from build123d import *

# Parameters (mm, degrees)
SKETCH1_R                = 7.5
BOSS_EXTRUDE1_DEPTH      = 15
BOSS_EXTRUDE2_DEPTH      = 45
BOSS_EXTRUDE3_DEPTH      = 18
BOSS_EXTRUDE3_DEPTH_BACK = 15
CUT_EXTRUDE1_REACH       = 187.068
SKETCH2_R                = 4
CUT_EXTRUDE2_REACH       = 188.456
SKETCH3_R                = 5


with BuildPart() as part:
    # Sketch1 → Boss-Extrude1 (new, symmetric)
    with BuildSketch(Plane.XY):
        with BuildLine():
            Line((145, 15), (80, 15))
            Line((80, 15), (80, 0))
            Line((80, 0), (175, 0))
            Line((175, 0), (175, 31))
            ThreePointArc((175, 31), (160, 46), (145, 31))
            Line((145, 31), (145, 15))
        make_face()
        with Locations((160, 31)):
            Circle(SKETCH1_R, mode=Mode.SUBTRACT)
    extrude(amount=BOSS_EXTRUDE1_DEPTH, both=True)



with BuildPart() as body_2:
    # Sketch1_3 → Boss-Extrude2 (new, symmetric)
    with BuildSketch(Plane.XY):
        Polygon((65, 15), (0, 15), (0, -25), (16, -25), (16, 0), (80, 0), align=None)
    extrude(amount=BOSS_EXTRUDE2_DEPTH, both=True)


with BuildPart() as part_1:
    add(part.part)

    add(body_2.part)  # Boss-Extrude3 merges body 2
    # Sketch1_4 → Boss-Extrude3 (add, two sides: drawn at the far end of the back side and taken through both)
    with BuildSketch(Plane.XY.offset(-BOSS_EXTRUDE3_DEPTH_BACK)):
        Polygon((80, 15), (65, 15), (80, 0), align=None)
    extrude(amount=BOSS_EXTRUDE3_DEPTH + BOSS_EXTRUDE3_DEPTH_BACK)

    # Sketch2 → Cut-Extrude1 (cut, up to next)
    with BuildSketch(Plane(origin=(0, 15, 0), x_dir=(1, 0, 0), z_dir=(0, 1, 0)), mode=Mode.PRIVATE) as cut_extrude1_sk1:
        with Locations(Location((55, 0, 0), (0, 0, 180))):
            Circle(SKETCH2_R)
    cut_extrude1_tool1 = extrude(cut_extrude1_sk1.sketch, amount=-CUT_EXTRUDE1_REACH, mode=Mode.PRIVATE) & part_1.part
    # Sketch2 → Cut-Extrude1 (cut, up to next)
    with BuildSketch(Plane(origin=(0, 15, 0), x_dir=(1, 0, 0), z_dir=(0, 1, 0)), mode=Mode.PRIVATE) as cut_extrude1_sk2:
        with Locations(Location((30, 0, 0), (0, 0, 180))):
            Circle(SKETCH2_R)
    cut_extrude1_tool2 = extrude(cut_extrude1_sk2.sketch, amount=-CUT_EXTRUDE1_REACH, mode=Mode.PRIVATE) & part_1.part
    add(cut_extrude1_tool1.solids().sort_by_distance((55, 15, 0))[0], mode=Mode.SUBTRACT)
    add(cut_extrude1_tool2.solids().sort_by_distance((30, 15, 0))[0], mode=Mode.SUBTRACT)

    # Sketch3 → Cut-Extrude2 (cut, up to next)
    with BuildSketch(Plane.ZY, mode=Mode.PRIVATE) as cut_extrude2_sk1:
        with Locations(Location((35, -15, 0), (0, 0, 270))):
            Circle(SKETCH3_R)
    cut_extrude2_tool1 = extrude(cut_extrude2_sk1.sketch, amount=-CUT_EXTRUDE2_REACH, mode=Mode.PRIVATE) & part_1.part
    # Sketch3 → Cut-Extrude2 (cut, up to next)
    with BuildSketch(Plane.ZY, mode=Mode.PRIVATE) as cut_extrude2_sk2:
        with BuildLine():
            Line((45, -25), (45, -15))
            ThreePointArc((45, -15), (42.071067812, -22.071067812), (35, -25))
            Line((35, -25), (45, -25))
        make_face()
    cut_extrude2_tool2 = extrude(cut_extrude2_sk2.sketch, amount=-CUT_EXTRUDE2_REACH, mode=Mode.PRIVATE) & part_1.part
    # Sketch3 → Cut-Extrude2 (cut, up to next)
    with BuildSketch(Plane.ZY, mode=Mode.PRIVATE) as cut_extrude2_sk3:
        with Locations(Location((-35, -15, 0), (0, 0, 270))):
            Circle(SKETCH3_R)
    cut_extrude2_tool3 = extrude(cut_extrude2_sk3.sketch, amount=-CUT_EXTRUDE2_REACH, mode=Mode.PRIVATE) & part_1.part
    # Sketch3 → Cut-Extrude2 (cut, up to next)
    with BuildSketch(Plane.ZY, mode=Mode.PRIVATE) as cut_extrude2_sk4:
        with BuildLine():
            Line((-45, -25), (-35, -25))
            ThreePointArc((-35, -25), (-42.071067806, -22.071067818), (-45, -15.000000016))
            Line((-45, -15.000000016), (-45, -25))
        make_face()
    cut_extrude2_tool4 = extrude(cut_extrude2_sk4.sketch, amount=-CUT_EXTRUDE2_REACH, mode=Mode.PRIVATE) & part_1.part
    add(cut_extrude2_tool1.solids().sort_by_distance((0, -15, 35))[0], mode=Mode.SUBTRACT)
    add(cut_extrude2_tool2.solids().sort_by_distance((0, -22.766321, 42.766321))[0], mode=Mode.SUBTRACT)
    add(cut_extrude2_tool3.solids().sort_by_distance((0, -15, -35))[0], mode=Mode.SUBTRACT)
    add(cut_extrude2_tool4.solids().sort_by_distance((0, -22.766321, -42.766321))[0], mode=Mode.SUBTRACT)


solid = part_1.part
Build history of the part. All positions in model axes, mm. A direction names the side the tool comes from. Coordinates: 2 decimals unless noted, no trailing zeros. Write each loop counter-clockwise with the first axis right and the second up, starting at its lowest first coordinate (ties: lowest second). Pieces come first, ordered by that corner, then holes.
(1) 3-axis set-ups, long thin cutter, end or side, ignore diameter. For faces 1 (the flat face through (137, 13, 15)), 2 (the flat face through (73, 7, -30)), 3 (the flat face through (77, 0, 1)): which of +Z, -Z, +X, -X, +Y, -Y reach the whole face in a straight line?
(2) Cut at C-C on y = 9. List the corners of the cut face in (x, z).
(3) Cut at D-D on z = 13. List the corners of the cut face in (x, y).
(4) Cut at A-A on x = 55. List the corners of the cut face in (y, z).
(5) Cut at B-B on z = 0. List the corners of the cut face in (x, y).
(6) Drill centre lines: line 1 (Z direction, x = 7, y = -15); line 2 (Z direction, x = 55, y = 9); line 3 (Z direction, x = 99, y = 14). Where is each one in solid material? Low to high.
(7) Pin check, flat tips, straight feed: pin 1 Ø5 at (x, z) = (49.5, -8.5) entering from -Y; pin 2 Ø14 at (x, y) = (146, 31.5) entering from -Z; pin 3 Ø6 at (y, z) = (-15, 35) entering from +X; pin 4 Ø8 at (y, z) = (23, -1.5) entering from -X. Stop position of each tip, or through.
(8) Mould opens along X. For faces 4 (the flat face through (131, 13, -15)), 5 (the flat face through (0, -5, 1)), 6 (the cylindrical face through (166.93, 28.13, -0.21)) say: pulls with the +X half, pulls with the -X half, needs draft (parallel to the pull), parting line crosses it, or undercut.
Working result:
1. face 1: +Z, +X, +Y, -Y
1. face 2: -Z, +X, +Y
1. face 3: +Z, -Z, +X, -Y
2. outline: (0, -45) - (71, -45) - (71, -15) - (175, -15) - (175, 15) - (80, 15) - (80, 18) - (71, 18) - (71, 45) - (0, 45) - close; hole circle Ø8 at (30, 0); hole circle Ø8 at (55, 0)
3. outline: (0, -25) - (16, -25) - (16, 0) - (175, 0) - (175, 31) arc R15 ccw to (145, 31) - (145, 15) - (0, 15) - close; hole circle Ø15 at (160, 31)
4. outline: (0, -45) - (15, -45) - (15, -4) - (0, -4) - close; (0, 4) - (15, 4) - (15, 45) - (0, 45) - close
5. outline: (0, -25) - (16, -25) - (16, 0) - (26, 0) - (26, 15) - (0, 15) - close; (34, 0) - (51, 0) - (51, 15) - (34, 15) - close; (59, 0) - (175, 0) - (175, 31) arc R15 ccw to (145, 31) - (145, 15) - (59, 15) - close; hole circle Ø15 at (160, 31)
6. line 1: z = -45 to -40, -30 to 30, 40 to 45
6. line 2: z = -45 to -4, 4 to 45
6. line 3: z = -15 to 15
7. pin 1: stops at y = 0
7. pin 2: stops at z = -15
7. pin 3: passes through
7. pin 4: stops at x = 145
8. face 4: needs draft
8. face 5: pulls with the -X half
8. face 6: undercut
